Source: CAD feature listing. Evaluate the final solid. Frame: model axes, mm. A direction names the side the tool comes from. Give positions to 0.01 mm unless a question says otherwise; leave off trailing zeros. Write each loop counter-clockwise with the first axis right and the second up, starting at its lowest first coordinate (ties: lowest second). Pieces come first, ordered by that corner, then holes.
```python
from build123d import *

# Parameters (mm, degrees)
BODY_DEPTH               = 10
SKETCH3_W                = 16.2
SKETCH3_H                = 8
SKETCH7_R                = 3.2
REAR_MOUNTING_DEPTH      = 21.05
REAR_MOUNTING_DEPTH_BACK = 21.05
SKETCH8_R                = 2.4
HOLE_DEPTH               = 8.5
FILLET4_R                = 2


with BuildPart() as part:
    # Sketch1 → Body (new body)
    with BuildSketch(Plane.XY.offset(130.3)):
        with BuildLine():
            Line((20.05, 9), (17.6, 12.720551034))
            Line((17.6, 12.720551034), (17.6, 32.8))
            ThreePointArc((17.6, 32.8), (12.445079349, 45.245079349), (0, 50.4))
            ThreePointArc((0, 50.4), (-12.445079349, 45.245079349), (-17.6, 32.8))
            Line((-17.6, 32.8), (-17.6, 12.720551034))
            Line((-17.6, 12.720551034), (-20.05, 9))
            Line((-20.05, 9), (-20.05, 0))
            Line((-20.05, 0), (-20.05, -11.4))
            Line((-20.05, -11.4), (-11.588549493, -18.5))
            Line((-11.588549493, -18.5), (-7.016550666, -18.5))
            Line((-7.016550666, -18.5), (7.016550666, -18.5))
            Line((7.016550666, -18.5), (11.588549493, -18.5))
            Line((11.588549493, -18.5), (20.05, -11.4))
            Line((20.05, -11.4), (20.05, 0))
            Line((20.05, 0), (20.05, 9))
        make_face()
    extrude(amount=BODY_DEPTH)

    # Sketch3 → Motor-Body (revolve)
    with BuildSketch(Plane(origin=(0, 0, 0), x_dir=(0, 0, -1), z_dir=(1, 0, 0))):
        with Locations((-148.4, 4)):
            Rectangle(SKETCH3_W, SKETCH3_H)
    revolve(axis=Axis((0, 0, -96.607444662), (0, 0, 1)))

    # Sketch7 → Rear-Mounting (cut, two sides)
    with BuildSketch(Plane(origin=(0, 0, 0), x_dir=(0, 0, -1), z_dir=(1, 0, 0))) as rear_mounting_sk:
        with Locations((-148.4, 0)):
            Circle(SKETCH7_R)
    extrude(amount=REAR_MOUNTING_DEPTH, mode=Mode.SUBTRACT)
    extrude(rear_mounting_sk.sketch, amount=-REAR_MOUNTING_DEPTH_BACK, mode=Mode.SUBTRACT)

    # Sketch8 → Hole (cut)
    with BuildSketch(Plane.XY.offset(130.3)):
        with Locations((16, -9)):
            Circle(SKETCH8_R)
        with Locations((-16, -9)):
            Circle(SKETCH8_R)
        with Locations((-16, 9)):
            Circle(SKETCH8_R)
        with Locations((16, 9)):
            Circle(SKETCH8_R)
    extrude(amount=HOLE_DEPTH, mode=Mode.SUBTRACT)

    # Fillet4
    fillet4_edges = [part.edges().sort_by_distance(p)[0] for p in [
        (-17.6, 22.760275517, 140.3),
        (-18.825, 10.860275517, 140.3),
        (-20.05, -1.2, 140.3),
        (-15.819274746, -14.95, 140.3),
        (0, -18.5, 140.3),
        (15.819274746, -14.95, 140.3),
        (20.05, -1.2, 140.3),
        (0, 50.4, 140.3),
        (18.825, 10.860275517, 140.3),
        (17.6, 22.760275517, 140.3),
    ]]
    fillet(fillet4_edges, radius=FILLET4_R)


solid = part.part
```
1. Access query for faces 4 (the cylindrical face through (13.602, -8.894, 134.49)), 5 (the cylindrical face through (-17, 22.32, 139.73)), 6 (the flat face through (-17.6, 23, 134)), 7 (the flat face through (17.6, 23, 134)). Directions: +Z, -Z, +X, -X, +Y, -Y. A direction counts if a zero-diameter tool reaches every point of the face in a straight line with its end or side. Return the directions, or none.
2. Cut plane C-C, the plane z = 150.5. Return the cut outline in (x, y), then the cut area to 3 significant figures.
3. Cut plane B-B, the plane z = 136.75. Return the cut outline in (x, y), then the cut area to 3 significant figures.
4. Contact query for flat-ended pins moving along their axis: P1, Ø7.5, axis at y = 0, z = 148.4, coming from the +X side; P2, Ø4, axis at x = 16, y = 9, coming from the -Z side; P3, Ø6.5, axis at y = 23, z = 132.5, coming from the -X side. Output: stop coordinate, or through.
5. Cut plane A-A, the plane y = 0. Return the cut outline in (x, z).
6. Mould query, pull axis X, two halves, no side actions, for faces 1 (the cylindrical face through (0.16, -17.9, 139.73)), 2 (the flat face through (-16, -9, 138.8)), 3 (the flat face through (-18.8, 10.9, 134.2)). Classes: +X half, -X half, draft (parallel to the pull), parting line (faces both ways), or undercut.
7. Line query: L1, parallel to Y at x = 16, z = 136.75; L2, parallel to Z at x = -14, y = 14.5; L3, parallel to Z at x = 15.5, y = -10. Output: solid intervals per line, ascending.
8. Cut plane D-D, the plane z = 154.75. Return the cut outline in (x, y).
Response values:
1. face 4: -Z
1. face 5: +Z, -X, +Y
1. face 6: +Z, -Z, -X, +Y
1. face 7: +Z, -Z, +X, +Y
2. outline: (-7.63, -2.41) arc R8 ccw to (7.63, -2.41) - close; (-7.63, 2.41) - (7.63, 2.41) arc R8 ccw to start
2. area: 125 mm2
3. outline: (-20.05, -11.4) - (-11.59, -18.5) - (11.59, -18.5) - (20.05, -11.4) - (20.05, 9) - (17.6, 12.72) - (17.6, 32.8) arc R17.6 ccw to (-17.6, 32.8) - (-17.6, 12.72) - (-20.05, 9) - close; hole circle Ø4.8 at (-16, -9); hole circle Ø4.8 at (-16, 9); hole circle Ø4.8 at (16, -9); hole circle Ø4.8 at (16, 9)
3. area: 2,300 mm2
4. P1: stops at x = 8
4. P2: stops at z = 138.8
4. P3: stops at x = -17.6
5. outline: (-20.05, 130.3) - (20.05, 130.3) - (20.05, 138.3) arc R2 ccw to (18.05, 140.3) - (8, 140.3) - (8, 145.2) - (-8, 145.2) - (-8, 140.3) - (-18.05, 140.3) arc R2 ccw to (-20.05, 138.3) - close; (-8, 151.6) - (8, 151.6) - (8, 156.5) - (-8, 156.5) - close
6. face 1: draft
6. face 2: undercut
6. face 3: -X half
7. L1: y = -14.8 to -11.4, -6.6 to 6.6, 11.4 to 40.13
7. L2: z = 130.3 to 140.3
7. L3: z = 138.8 to 140.3
8. outline: circle Ø16 at (0, 0)
